For this review, take the finished solid that the model builds, in its own axes (mm). A direction names the side the tool comes from. Coordinates: 2 decimals unless noted, no trailing zeros. Write each loop counter-clockwise with the first axis right and the second up, starting at its lowest first coordinate (ties: lowest second). Pieces come first, ordered by that corner, then holes. Notation, with made-up numbers: M -30,2.5 L 9,2.5 A29 cw 9,30.5 Z; hole C 0,9.25 d1. An arc over 180 degrees is marked long. Return JSON: item names as keys, results as strings.
```python
from build123d import *

# Parameters (mm, degrees)
SKETCH1_R             = 40
BOSS_EXTRUDE1_DEPTH   = 60
BOSS_EXTRUDE1_2_DEPTH = 60
BOSS_EXTRUDE3_START   = -3.447986
SKETCH5_W             = 40
SKETCH5_H             = 60
BOSS_EXTRUDE3_DEPTH   = 207.084974
SKETCH3_R             = 6
CUT_EXTRUDE3_DEPTH    = 10
SKETCH4_R             = 6
BOSS_EXTRUDE4_DEPTH   = 10
SKETCH6_R             = 30
CUT_EXTRUDE4_DEPTH    = 10


with BuildPart() as part:
    # Sketch1 → Boss-Extrude1 (new body)
    with BuildSketch(Plane.XY):
        Circle(SKETCH1_R)
    extrude(amount=BOSS_EXTRUDE1_DEPTH)



with BuildPart() as body_2:
    # Sketch1 → Boss-Extrude1 2 (new body)
    with BuildSketch(Plane.XY):
        with Locations((260, 0)):
            Circle(SKETCH1_R)
    extrude(amount=BOSS_EXTRUDE1_2_DEPTH)


with BuildPart() as part_1:
    add(part.part)

    add(body_2.part)  # Boss-Extrude3 merges body 2
    # Sketch5 → Boss-Extrude3 (add)
    with BuildSketch(Plane.ZY.offset(-230.094500915).offset(BOSS_EXTRUDE3_START)):
        with Locations((30, 0)):
            Rectangle(SKETCH5_W, SKETCH5_H)
    extrude(amount=BOSS_EXTRUDE3_DEPTH)

    # Sketch3 → Cut-Extrude3 (cut)
    with BuildSketch(Plane(origin=(0, 0, 0), x_dir=(-1, 0, 0), z_dir=(0, 0, -1))):
        Circle(SKETCH3_R)
    extrude(amount=-CUT_EXTRUDE3_DEPTH, mode=Mode.SUBTRACT)

    # Sketch4 → Boss-Extrude4 (add)
    with BuildSketch(Plane(origin=(0, 0, 0), x_dir=(-1, 0, 0), z_dir=(0, 0, -1))):
        with Locations((-260, 0)):
            Circle(SKETCH4_R)
    extrude(amount=BOSS_EXTRUDE4_DEPTH)

    # Sketch6 → Cut-Extrude4 (cut)
    with BuildSketch(Plane.XY.offset(60)):
        Circle(SKETCH6_R)
        with Locations((260, 0)):
            Circle(SKETCH6_R)
    extrude(amount=-CUT_EXTRUDE4_DEPTH, mode=Mode.SUBTRACT)


solid = part_1.part
```
1. We need section C-C (x = 260). State the section outline as (y, z) points.
Checks:
{"outline": "M -40,0 L -6,0 L -6,-10 L 6,-10 L 6,0 L 40,0 L 40,60 L 30,60 L 30,50 L -30,50 L -30,60 L -40,60 Z"}
2. We need section B-B (y = 0). State the section outline as (x, z) points, plus the area to 3 significant figures.
Checks:
{"outline": "M -40,0 L -6,0 L -6,10 L 6,10 L 6,0 L 40,0 L 40,10 L 220,10 L 220,0 L 254,0 L 254,-10 L 266,-10 L 266,0 L 300,0 L 300,60 L 290,60 L 290,50 L 230,50 L 230,60 L 220,60 L 220,50 L 40,50 L 40,60 L 30,60 L 30,50 L -30,50 L -30,60 L -40,60 Z", "area": "15,600 mm2"}
3. Wall thickness on L1, parallel to Y at x = 0, z = 7; L2, parallel to Y at x = 260, z = 57; L3, parallel to Z at x = 153.5, y = -4.5: over which ranges is each line inside the solid? List them lowest first. Write a range as from..to.
Checks:
{"L1": "-40..-6, 6..40", "L2": "-40..-30, 30..40", "L3": "10..50"}
4. We need section A-A (z = 4.5). State the section outline as (x, y) points.
Checks:
{"outline": "C 0,0 d80; C 260,0 d80; hole C 0,0 d12"}
5. For faces 4 (the face through (131, 30, 30)), 5 (the face through (260, 0, 50)), 6 (the face through (0, 0, 10)), 7 (the face through (8, 1, 0)), list the 3-axis set-ups (+Z, -Z, +X, -X, +Y, -Y) from which the entire face can be reached by the end or side of a thin tool; tool diameter is ignored.
Checks:
{"face 4": "+Z, -Z, +Y", "face 5": "+Z", "face 6": "-Z", "face 7": "-Z, -X, +Y, -Y"}
6. Clearance check with flat-ended pins moving along their axes: pin 1 Ø5 at (y, z) = (-3.5, 0.5) entering from -X; pin 2 Ø12 at (x, y) = (99, -18.5) entering from -Z; pin 3 Ø4 at (y, z) = (30.5, 4.5) entering from +X; pin 4 Ø1 at (x, z) = (119.5, 8) entering from -Y. State where each tip first meets the part, or that it passes through.
Checks:
{"pin 1": "x = -39.99", "pin 2": "z = 10", "pin 3": "x = 288.07", "pin 4": "through"}
7. Draft analysis for pull direction X (two halves, no side actions). For faces 1 (the face through (254.277, 1.802, -4.93)), 2 (the face through (266, 30, 60)), 3 (the face through (131, 0, 50)), state which applies: +X half, -X half, draft (parallel to the pull), parting line (faces both ways), or undercut.
Checks:
{"face 1": "parting line", "face 2": "draft", "face 3": "undercut"}
8. We need section D-D (y = 35). State the section outline as (x, z) points.
Checks:
{"outline": "M -19.36,0 L 19.36,0 L 19.36,60 L -19.36,60 Z; M 240.64,0 L 279.36,0 L 279.36,60 L 240.64,60 Z"}
